```python
from build123d import *

# Parameters (mm, degrees)
F0_R          = 44.45
F0_R_2        = 2.5
F0_R_3        = 11.1125
F0_R_4        = 7.9375
F1_DEPTH      = 6.35
F2_DEPTH      = 38.1
F3_R          = 2.5
F4_DEPTH      = 44.451
F4_DEPTH_BACK = 44.451
F5_SIZE       = 1.27
F6_SIZE       = 2.54
F7_R          = 1.524


with BuildPart() as f1:
    # F0 (on Top) → F1 (new body)
    with BuildSketch(Plane.XY):
        Circle(F0_R)
        with Locations((-20.5283999363, -28.2549185285)):
            Circle(F0_R_2, mode=Mode.SUBTRACT)
        with Locations((20.5283999363, -28.2549185285)):
            Circle(F0_R_2, mode=Mode.SUBTRACT)
        with Locations((-33.2156488316, 10.7924185285)):
            Circle(F0_R_2, mode=Mode.SUBTRACT)
        Circle(F0_R_3, mode=Mode.SUBTRACT)
        with Locations((33.2156488316, 10.7924185285)):
            Circle(F0_R_2, mode=Mode.SUBTRACT)
        with Locations((0, 34.925)):
            Circle(F0_R_2, mode=Mode.SUBTRACT)
        Circle(F0_R_3)
        Circle(F0_R_4, mode=Mode.SUBTRACT)
    extrude(amount=F1_DEPTH)

    # F0 (on Top) → F2 (join)
    with BuildSketch(Plane.XY):
        Circle(F0_R_3)
        Circle(F0_R_4, mode=Mode.SUBTRACT)
    extrude(amount=F2_DEPTH)

    # F3 (on Front) → F4 (cut, two sides)
    with BuildSketch(Plane.XZ) as f4_sk:
        with Locations((0, 12.7)):
            Circle(F3_R)
        with Locations((0, 28.575)):
            Circle(F3_R)
    extrude(amount=-F4_DEPTH, mode=Mode.SUBTRACT)
    extrude(f4_sk.sketch, amount=F4_DEPTH_BACK, mode=Mode.SUBTRACT)

    # F5
    f5_edges = [f1.edges().sort_by_distance(p)[0] for p in [
        (-7.9375, 0, 38.1),
        (-7.9375, 0, 0),
        (-44.45, 0, 6.35),
    ]]
    chamfer(f5_edges, length=F5_SIZE)

    # F6
    f6_edges = [f1.edges().sort_by_distance(p)[0] for p in [
        (-11.1125, 0, 6.35),
    ]]
    chamfer(f6_edges, length=F6_SIZE)

    # F7
    f7_edges = [f1.edges().sort_by_distance(p)[0] for p in [
        (-11.1125, 0, 8.89),
        (-13.6525, 0, 6.35),
    ]]
    fillet(f7_edges, radius=F7_R)


solid = f1.part
```
The model under review builds one solid part; all positions refer to its coordinate system, in mm. A direction names the side the tool comes from. Round coordinates to 2 decimals unless told otherwise and drop trailing zeros. Loops run counter-clockwise (first coordinate to the right, second up) from the corner with the lowest first, then second, coordinate; pieces in that order, holes last.
Item 1: Clearance check with flat-ended pins moving along their axes: pin 1 Ø8 at (x, y) = (8.5, 35.5) entering from +Z; pin 2 Ø6 at (x, z) = (0, 28.575) entering from +Y; pin 3 Ø3 at (x, z) = (-10.5, 26.5) entering from -Y. State where each tip first meets the part, or that it passes through.
Determined:
pin 1: stops at z = 6.35
pin 2: stops at y = 11.11
pin 3: stops at y = -6.52
Item 2: Take a section at A-A (z = 3.5). Give the number of separate pieces and of enclosed holes in the cut face, then the cut area to 3 significant figures.
Determined:
separate pieces: 1
enclosed holes: 6
area: 5,910 mm2
Item 3: Mouldability with a two-part tool opening along Y and no side actions: class faces 3 (the face through (20, -30.7, 3.1)), 4 (the face through (-2.41, -10.85, 23.61)), 5 (the face through (-7, 7, 38.1)) as released by +Y, released by -Y, zero draft, split by the parting line, or undercut.
Determined:
face 3: undercut
face 4: split by the parting line
face 5: zero draft
Item 4: For faces 1 (the face through (-35.713, 10.902, 3.131)), 2 (the face through (19, 1, 6.35)), list the 3-axis set-ups (+Z, -Z, +X, -X, +Y, -Y) from which the entire face can be reached by the end or side of a thin tool; tool diameter is ignored.
Determined:
face 1: +Z, -Z
face 2: +Z
Item 5: Take a section at B-B (z = 23). Write out the cut boundary in (x, y) (1 decimal), then the cut area to 3 significant figures.
Determined:
outline: circle Ø22.2 at (0, 0); hole circle Ø15.9 at (0, 0)
area: 190 mm2
Item 6: For line 1 (Z direction, x = 0, y = 9.2) (1 decimal); line 2 (Y direction, x = 0, z = 18); line 3 (Z direction, x = 18.5, y = -18), list the stretches that pass through material, from the lowest coordinate up.
Determined:
line 1: z = 0 to 10.2, 15.2 to 26.1, 31.1 to 38.1
line 2: y = -11.11 to -7.94, 7.94 to 11.11
line 3: z = 0 to 6.35
Item 7: Take a section at C-C (z = 12.7). Write out the cut boundary in (x, y) (1 decimal), then the cut area to 3 significant figures.
Determined:
outline: (-2.5, -10.8) - (-2.5, -7.5) arc R7.9 cw to (-2.5, 7.5) - (-2.5, 10.8) arc R11.1 ccw to start; (2.5, -10.8) arc R11.1 ccw to (2.5, 10.8) - (2.5, 7.5) arc R7.9 cw to (2.5, -7.5) - close
area: 158 mm2
